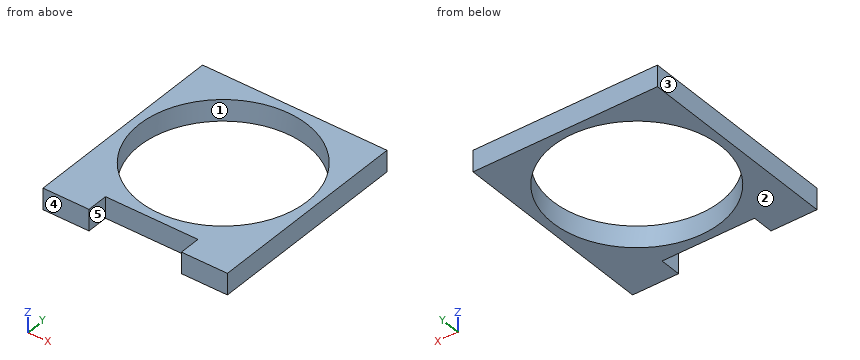
from build123d import *

# Parameters (mm, degrees)
BOSS_EXTRUDE1_DEPTH     = 6.35
CUT_EXTRUDE1_DEPTH      = 79.123725091
CUT_EXTRUDE1_DEPTH_BACK = 79.123725091
SKETCH3_R               = 25.000000038


with BuildPart() as part:
    # Sketch2 → Boss-Extrude1 (new body)
    with BuildSketch(Plane.XY):
        Polygon((13.716, 0), (41.283999982, 0), (41.283999982, -6.35), (54.999999982, -6.35), (54.999999982, 0), (54.999999982, 55.118), (0, 55.118), (0, 0), (0, -6.35), (13.716, -6.35), align=None)
    extrude(amount=BOSS_EXTRUDE1_DEPTH)

    # Sketch3 → Cut-Extrude1 (cut, two sides: drawn at the far end of the back side and taken through both)
    with BuildSketch(Plane.XY.offset(6.35).offset(-CUT_EXTRUDE1_DEPTH_BACK)):
        with Locations((27.499999991, 27.559)):
            Circle(SKETCH3_R)
    extrude(amount=CUT_EXTRUDE1_DEPTH + CUT_EXTRUDE1_DEPTH_BACK, mode=Mode.SUBTRACT)


solid = part.part
Source: CAD feature listing. Evaluate the final solid. Frame: model axes, mm. Face numbers are marked on the shaded views. A direction names the side the tool comes from. Round coordinates to 2 decimals unless told otherwise and drop trailing zeros. Order: outer loops, then holes, each group sorted by start corner. A loop starts at its lowest first (then second) coordinate and runs counter-clockwise, first axis right, second up. Notation, with made-up numbers: (37, -12) - (48, -12) arc R30 cw to (48, 15) - close; hole circle Ø8 at (35.25, 47.5). An arc over 180 degrees is marked (long way). Use a Markdown table: item, result. Add a question column.
1. Section query B-B (y = 9). Return the cut outline in (x, z).
2. Mould query, pull axis X, two halves, no side actions, for the marked faces 1, 2 and 3. Classes: +X half, -X half, draft (parallel to the pull), parting line (faces both ways), or undercut.
3. Line query: probe 1 along Y at (x, z) = (27.5, 3.25); probe 2 along X at (y, z) = (12, 4.25); probe 3 along Y at (x, z) = (49.5, 2.75). Output: solid intervals per line, ascending.
4. Section query A-A (x = 27.5). Return the cut outline in (y, z), then the cut area to 3 significant figures.
5. Section query C-C (z = 4.5). Return the cut outline in (x, y).
6. First-contact query: pin 1 (1 mm diameter, centred on x = 17, z = 2, fed in from -Y); pin 2 (2 mm diameter, centred on x = 21, y = 3.5, fed in from -Z). Flat tips, straight axial feed; report the tip coordinate or a pass-through.
7. Set-up query: the marked faces 4 and 5. Return all of +Z, -Z, +X, -X, +Y, -Y with unobstructed straight access to the full face (end or side cutting, diameter ignored); none if empty.
Derived:
| question | item | result |
|---|---|---|
| 1 | outline | (0, 0) - (10.75, 0) - (10.75, 6.35) - (0, 6.35) - close; (44.25, 0) - (55, 0) - (55, 6.35) - (44.25, 6.35) - close |
| 2 | face 1 | undercut |
| 2 | face 2 | draft |
| 2 | face 3 | -X half |
| 3 | probe 1 | 0 to 2.56, 52.56 to 55.12 |
| 3 | probe 2 | 0 to 7.93, 47.07 to 55 |
| 3 | probe 3 | -6.35 to 15.68, 39.43 to 55.12 |
| 4 | outline | (0, 0) - (2.56, 0) - (2.56, 6.35) - (0, 6.35) - close; (52.56, 0) - (55.12, 0) - (55.12, 6.35) - (52.56, 6.35) - close |
| 4 | area | 32.5 mm2 |
| 5 | outline | (0, -6.35) - (13.72, -6.35) - (13.72, 0) - (41.28, 0) - (41.28, -6.35) - (55, -6.35) - (55, 55.12) - (0, 55.12) - close; hole circle Ø50 at (27.5, 27.56) |
| 6 | pin 1 | y = 0 |
| 6 | pin 2 | z = 0 |
| 7 | face 4 | +Z, -Z, +X, -X, -Y |
| 7 | face 5 | +Z, -Z, -Y |
